Autodesk Inventor part; units mm, degrees
ref_plane "YZ Plane" through (0, 0, 0) normal (1, 0, 0) x (0, 1, 0)
ref_plane "XZ Plane" through (0, 0, 0) normal (0, 1, 0) x (-1, 0, 0)
ref_plane "XY Plane" through (0, 0, 0) normal (0, 0, 1) x (1, 0, 0)
sketch "Skizze1" plane through (0, 0, 0) normal (1, 0, 0) x (0, 1, 0)
  line L0 (-42.5, 127.5) -> (42.5, 127.5)
  line L1 (42.5, 127.5) -> (42.5, -127.5)
  line L2 (42.5, -127.5) -> (-42.5, -127.5)
  line L3 (-42.5, -127.5) -> (-42.5, 127.5)
  line L4 (-42.5, 127.5) -> (42.5, -127.5) construction
  line L5 (42.5, 127.5) -> (-42.5, -127.5) construction
  point P0 (0, 0)
  dimension "d0" = 85
  dimension "d1" = 255
extrude "Extrusion1" add sketch "Skizze1" along normal blind 10
sketch "Skizze2" plane through (10, 0, 0) normal (1, 0, 0) x (0, 0, -1)
  line L0 (-127.5, 42.5) -> (-127.5, -42.5)
  line L1 (127.5, -42.5) -> (127.5, 42.5)
  line L2 (127.5, 42.5) -> (-127.5, 42.5)
  point P0 (0, 0)
  point P1 (-107.5, -7.4)
  point P2 (-2.5, -7.4)
  point P3 (102.5, -7.4)
  dimension "d4" = 20
  dimension "d5" = 25
  dimension "d6" = 105
  dimension "d7" = 49.9
  dimension "d8" = 49.9
  dimension "d9" = 49.9
hole "Bohrung1" at (10, -7.4, 107.5) at (10, -7.4, 2.5) at (10, -7.4, -102.5) direction (-1, 0, 0) diameter 3.242 end through all counterbore diameter 7 counterbore depth 4
sketch "Skizze3" plane through (0, 42.5, 127.5) normal (0, 1, 0) x (1, 0, 0)
  line L0 (0, 0) -> (10, 0)
  line L1 (5, 0) -> (5, 250)
  line L2 (0, 255) -> (10, 255)
  point P0 (0, 127.5)
  point P1 (5, 20)
  point P2 (5, 125)
  point P3 (5, 230)
  point P4 (5, 255)
  dimension "d17" = 20
  dimension "d18" = 25
  dimension "d19" = 105
hole "Bohrung2" at (5, 42.5, 107.5) at (5, 42.5, 2.5) at (5, 42.5, -102.5) direction (0, -1, 0) diameter 3.242 depth 11.8 tip angle 118
mirror "Spiegeln1" about plane through (0, 0, 0) normal (0, 1, 0) of "Bohrung2"
properties part number "ER_Wand_1"
Input: part model. Units: mm. Frame: model coordinates. A direction names the side the tool comes from. Coordinates: 2 decimals unless noted, no trailing zeros.
(1) Pull-direction query (Z, two-part tool) for faces 1 (the face through (5, -1, 127.5)), 2 (the face through (7.972, -6.059, 104.267)), 3 (the face through (7.972, -6.059, -105.733)), 4 (the face through (3, 42.5, 2)); classes: released by +Z, released by -Z, zero draft, split by the parting line, or undercut.
(2) Set-up query: faces 5 (the face through (7.972, -4.295, 0.885)), 6 (the face through (5, -42.5, -2)). Return all of +Z, -Z, +X, -X, +Y, -Y with unobstructed straight access to the full face (end or side cutting, diameter ignored); none if empty.
(3) First-contact query: pin 1 Ø3 at (x, z) = (5, -102.5) entering from -Y; pin 2 Ø1.9 at (x, z) = (5, 107.5) entering from -Y; pin 3 Ø5.5 at (y, z) = (-7.4, 107.5) entering from +X. Flat tips, straight axial feed; report the tip coordinate or a pass-through.
(4) Material intervals for probe 1 along Y at (x, z) = (1.45, 2.5); probe 2 along X at (y, z) = (40, 2.5); probe 3 along Y at (x, z) = (6.9, 2.5), sorted ascending.
Data:
1. face 1: released by +Z
1. face 2: undercut
1. face 3: undercut
1. face 4: zero draft
2. face 5: +X
2. face 6: +Z, -Z, +X, -X, -Y
3. pin 1: stops at y = -30.63
3. pin 2: stops at y = -30.3
3. pin 3: stops at x = 6
4. probe 1: y = -42.5 to -9.02, -5.78 to 42.5
4. probe 2: x = 0 to 3.38, 6.62 to 10
4. probe 3: y = -42.5 to -10.9, -3.9 to 42.5
